For this review, take the finished solid that the model builds, in its own axes (mm). A direction names the side the tool comes from. Round coordinates to 2 decimals unless told otherwise and drop trailing zeros. Loops run counter-clockwise (first coordinate to the right, second up) from the corner with the lowest first, then second, coordinate; pieces in that order, holes last.
1. Consider section C-C on y = 6.25. State the section outline as (x, z) points, then the cut area to 3 significant figures.
2. Consider section D-D on z = 0.75. State the section outline as (x, y) points.
3. Draft analysis for pull direction Z (two halves, no side actions). For faces 4 (the flat face through (0, 11, -7.82)), 5 (the flat face through (0, 5, 5.08)), 6 (the flat face through (-2.5, 12, 1)), state which applies: released by +Z, released by -Z, zero draft, split by the parting line, or undercut.
4. Tool access review of faces 1 (the flat face through (0, 12, 4)), 2 (the flat face through (3.81, 5, -6)), 3 (the flat face through (0, 5, -7.62)): name each direction out of +Z, -Z, +X, -X, +Y, -Y from which nothing blocks a thin tool from reaching the whole face with its end or side.
5. To check wall thickness, follow line 1 along X through (y, z) = (9.25, 6.35); line 2 along Z through (x, y) = (0, 3.75); line 3 along Y through (x, z) = (-3, 0.5). State the ranges of each line that lie inside material, in increasing order.
6. Consider section A-A on z = -6.35. State how many separate pieces and enclosed holes the cut face has, then the cut area to 3 significant figures.
7. Clearance check with flat-ended pins moving along their axes: pin 1 Ø2 at (y, z) = (4.5, 6.5) entering from +X; pin 2 Ø3 at (y, z) = (7, 7) entering from -X; pin 3 Ø2 at (x, z) = (-3, 6.5) entering from +Y; pin 4 Ø2 at (x, z) = (0, -1.5) entering from +Y. State where each tip first meets the part, or that it passes through.
Autodesk Inventor part; units mm, degrees
ref_plane "YZ Plane" through (0, 0, 0) normal (1, 0, 0) x (0, 1, 0)
ref_plane "XZ Plane" through (0, 0, 0) normal (0, 1, 0) x (-1, 0, 0)
ref_plane "XY Plane" through (0, 0, 0) normal (0, 0, 1) x (1, 0, 0)
sketch "スケッチ1" plane through (0, 0, 0) normal (0, 1, 0) x (-1, 0, 0)
  line L0 (3.81, -5.08) -> (-3.81, -5.08)
  line L1 (-3.81, -5.08) -> (-3.81, -7.62)
  line L2 (-3.81, -7.62) -> (3.81, -7.62)
  line L3 (3.81, -7.62) -> (3.81, -5.08)
  line L4 (3.81, 7.62) -> (-3.81, 7.62)
  line L5 (-3.81, 7.62) -> (-3.81, 5.08)
  line L6 (-3.81, 5.08) -> (3.81, 5.08)
  line L7 (3.81, 5.08) -> (3.81, 7.62)
  line L8 (5.334, 0) -> (-5.334, 0)
  point P0 (0, 0)
  point P1 (0, 7.62)
  point P2 (3.81, 6.35)
  point P3 (3.81, -6.35)
  point P4 (-5.334, 0)
  dimension "d0" = 7.62
  dimension "d1" = 2.54
  dimension "d2" = 12.7
extrude "押し出し1" add sketch "スケッチ1" along normal blind 10
sketch "スケッチ2" plane through (0, 10, 0) normal (0, 1, 0) x (1, 0, 0)
  line L0 (-4.01, -7.82) -> (4.01, -7.82)
  line L1 (4.01, -7.82) -> (4.01, 7.82)
  line L2 (4.01, 7.82) -> (-4.01, 7.82)
  line L3 (-4.01, 7.82) -> (-4.01, -7.82)
  line L4 (-3.81, -5.08) -> (-3.81, -7.62)
  line L5 (-3.81, -7.62) -> (3.81, -7.62)
  point P0 (0, 0)
  point P1 (0, -7.82)
  point P2 (-4.01, 0)
  dimension "d7" = 0.2
  dimension "d8" = 0.2
extrude "押し出し2" add sketch "スケッチ2" along normal blind 1.5
sketch "スケッチ3" plane through (0, 11.5, 0) normal (0, 1, 0) x (1, 0, 0)
  line L0 (3.81, -7.62) -> (3.81, -5.08)
  line L1 (-3.81, -7.62) -> (3.81, -7.62)
  line L2 (-3.81, -5.08) -> (-3.81, -7.62)
  line L3 (3.81, -5.08) -> (-3.81, -5.08)
  line L4 (3.81, 5.08) -> (3.81, 7.62)
  line L5 (-3.81, 5.08) -> (3.81, 5.08)
  line L6 (-3.81, 7.62) -> (-3.81, 5.08)
  line L7 (3.81, 7.62) -> (-3.81, 7.62)
  circle A0 centre (-2.54, -6.35) radius 1
  line L8 (-3.81, -5.08) -> (-3.81, -7.62)
  circle A1 centre (0, -6.35) radius 1
  circle A2 centre (2.54, -6.35) radius 1
  line L9 (-5.614, 0) -> (5.614, 0)
  circle A3 centre (-2.54, 6.35) radius 1
  line L10 (-3.81, 5.08) -> (-3.81, 7.62)
  circle A4 centre (0, 6.35) radius 1
  circle A5 centre (2.54, 6.35) radius 1
  circle A6 centre (-2.54, -6.35) radius 0.5
  circle A7 centre (0, -6.35) radius 0.5
  circle A8 centre (2.54, -6.35) radius 0.5
  circle A9 centre (-2.54, 6.35) radius 0.5
  circle A10 centre (0, 6.35) radius 0.5
  circle A11 centre (2.54, 6.35) radius 0.5
  line L11 (-2.5, -4) -> (2.5, -4)
  line L12 (2.5, -4) -> (2.5, 1)
  line L13 (2.5, 1) -> (-2.5, 1)
  line L14 (-2.5, 1) -> (-2.5, -4)
  line L15 (-1, 1) -> (1, 1)
  line L16 (1, 1) -> (1, 3)
  line L17 (1, 3) -> (-1, 3)
  line L18 (-1, 3) -> (-1, 1)
  point P0 (0.6683, -5.6061)
  point P1 (-3.81, -6.35)
  point P2 (-3.81, -6.35)
  point P3 (0, 0)
  point P4 (0.6683, 5.6061)
  point P5 (-3.81, 6.35)
  point P6 (-3.81, 6.35)
  point P7 (0, 1)
  point P8 (0, 3)
  dimension "d9" = 2
  dimension "d10" = 2.54
  dimension "d11" = 2.54
  dimension "d12" = 1
  dimension "d13" = 1
  dimension "d14" = 1
  dimension "d15" = 1
  dimension "d16" = 1
  dimension "d17" = 1
  dimension "d18" = 1
  dimension "d19" = 5
  dimension "d20" = 5
  dimension "d21" = 2
extrude "押し出し3" cut sketch "スケッチ3" against normal through all contours A6 | A7 | A8 | A9 | A10 | A11
extrude "押し出し4" cut sketch "スケッチ3" against normal blind 0.05 contours A0 | A1 | A2 | A3 | A4 | A5
extrude "押し出し5" add sketch "スケッチ3" along normal blind 1.5 contours L14 L13 L12 L9 | L9 L12 L11 L14
extrude "押し出し6" add sketch "スケッチ3" along normal blind 0.5 contours L18 L17 L16 L13
properties part number "TPS61230A"
Resolved:
1. outline: (-3.81, -7.62) - (3.81, -7.62) - (3.81, -5.08) - (-3.81, -5.08) - close; (-3.81, 5.08) - (3.81, 5.08) - (3.81, 7.62) - (-3.81, 7.62) - close; hole circle Ø1 at (-2.54, -6.35); hole circle Ø1 at (-2.54, 6.35); hole circle Ø1 at (0, -6.35); hole circle Ø1 at (0, 6.35); hole circle Ø1 at (2.54, -6.35); hole circle Ø1 at (2.54, 6.35)
1. area: 34.0 mm2
2. outline: (-4.01, 10) - (4.01, 10) - (4.01, 11.5) - (2.5, 11.5) - (2.5, 13) - (-2.5, 13) - (-2.5, 11.5) - (-4.01, 11.5) - close
3. face 4: released by -Z
3. face 5: undercut
3. face 6: zero draft
4. face 1: +Z, +X, -X, +Y
4. face 2: +Z, -Z, +X, -Y
4. face 3: -Z, +X, -X, -Y
5. line 1: x = -3.81 to -3.04, -2.04 to -0.5, 0.5 to 2.04, 3.04 to 3.81
5. line 2: z = -7.62 to -6.85, -5.85 to -5.08, 5.08 to 5.85, 6.85 to 7.62
5. line 3: y = 10 to 11.5
6. separate pieces: 4
6. enclosed holes: 0
6. area: 53.6 mm2
7. pin 1: stops at x = 3.81
7. pin 2: stops at x = -3.81
7. pin 3: stops at y = 11.5
7. pin 4: stops at y = 13
